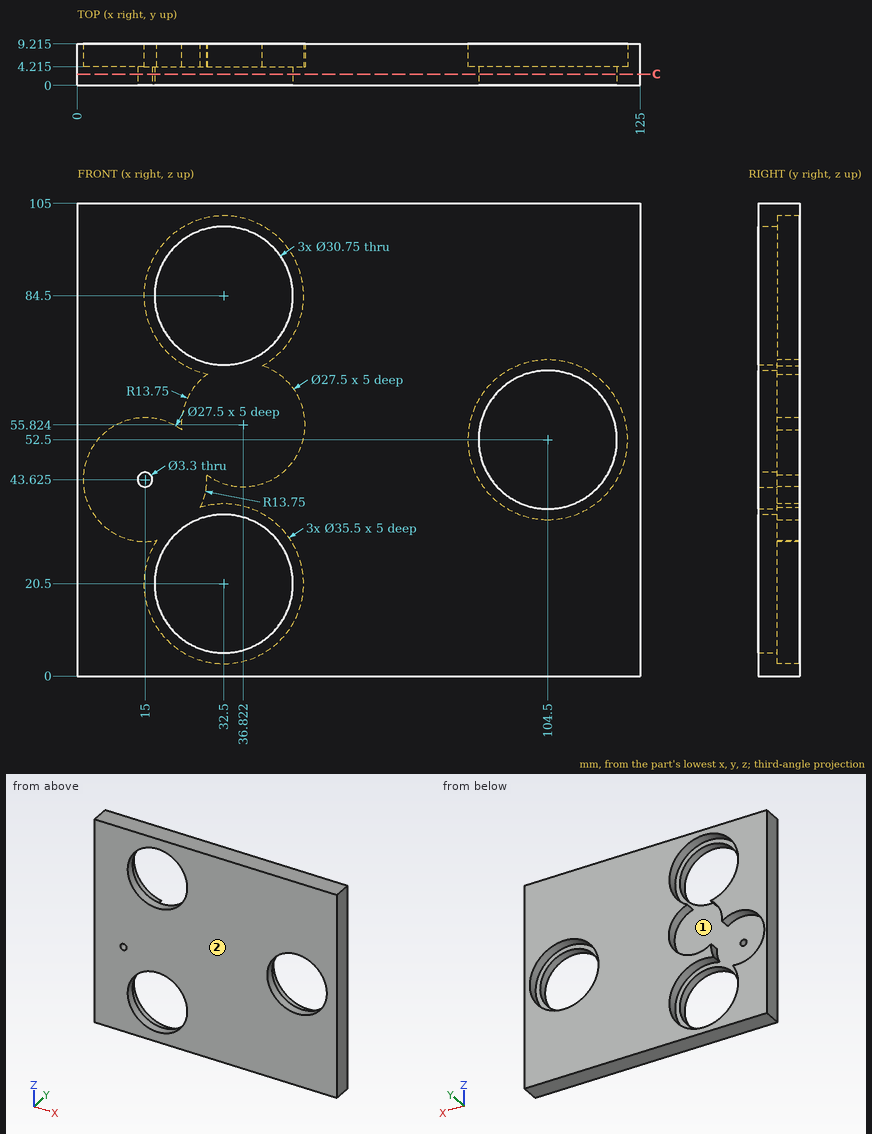
The figure shows three views and two pictorial views of one solid part (mm, origin at its lowest corner). Answer the questions. Round coordinates to 2 decimals unless told otherwise and drop trailing zeros. Answer as a JSON object with one key per item and string values. Group by question number.
Q1. Straight lines are drawn through the part: line 1 along X through (y, z) = (7.75, 54.5) (1 decimal); line 2 along Z through (x, y) = (29, 3.5); line 3 along X through (y, z) = (5.25, 20). For each, find the intervals that lie inside material, in ascending order.
Q2. Determine the mould class of the marked faces 1 and 2 for opening direction Z: pulls with the +Z half, pulls with the -Z half, needs draft (parallel to the pull), parting line crosses it, or undercut.
Q3. Each of these flat-tipped pins is pushed along its axis until it touches: pin 1 Ø21.5 at (x, z) = (32.5, 20.5) entering from +Y; pin 2 Ø1.5 at (x, z) = (59, 12.5) entering from -Y; pin 3 Ø16.5 at (x, z) = (36.82, 55.82) entering from +Y (3 decimals). Where does it stop, or does it pass through?
Q4. Section C-C (y = 2.5) is taken. Count the separate pieces of the cut face and the enclosed holes in it, plus the area to 3 significant figures.
Check values:
{
 "1": {"line 1": "0 to 6.6, 50.5 to 86.9, 122.1 to 125", "line 2": "0 to 5.53, 35.47 to 69.53, 99.47 to 105", "line 3": "0 to 14.76, 50.24 to 125"},
 "2": {"face 1": "undercut", "face 2": "needs draft"},
 "3": {"pin 1": "through", "pin 2": "y = 0", "pin 3": "y = 4.215"},
 "4": {"separate pieces": "1", "enclosed holes": "4", "area": "10,900 mm^2"}
}
